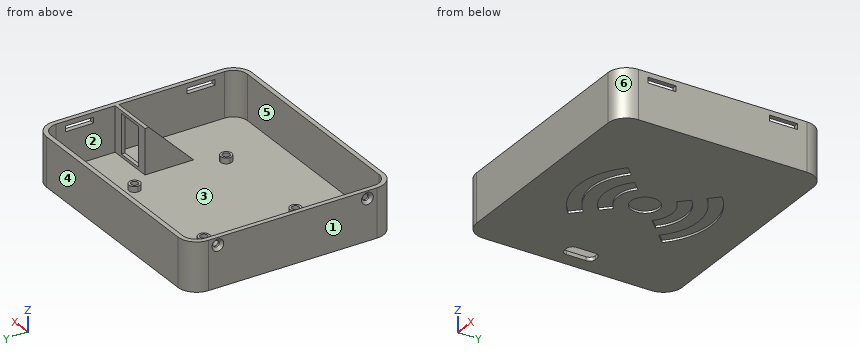
from build123d import *

# Parameters (mm, degrees)
P_IDAT_VYSUNUT_M1_DEPTH                           = 2
P_IDAT_VYSUNUT_M2_DEPTH                           = 24
SKICA6_R                                          = 3
P_IDAT_VYSUNUT_M3_DEPTH                           = 3
D_RY_PRO_KOL_K_VELIKOST_MM1_D                     = 3.8
D_RY_PRO_KOL_K_VELIKOST_MM1_DEPTH                 = 3.8
ODEBRAT_VYSUNUT_M1_DEPTH                          = 3
SKICA12_W                                         = 24
SKICA12_H                                         = 2
P_IDAT_VYSUNUT_M4_DEPTH                           = 25
P_IDAT_VYSUNUT_M5_DEPTH                           = 2
SKICA14_W                                         = 7.25
SKICA14_H                                         = 10.5
ODEBRAT_VYSUNUT_M2_DEPTH                          = 9.212713479
V_LCOV_ZAHLOUBEN_PRO_M3_ROUBY_S_PLOCH_D           = 3.4
V_LCOV_ZAHLOUBEN_PRO_M3_ROUBY_S_PLOCH_DEPTH       = 3.8
V_LCOV_ZAHLOUBEN_PRO_M3_ROUBY_S_PLOCH_CSINK_D     = 6.3
V_LCOV_ZAHLOUBEN_PRO_M3_ROUBY_S_PLOCH_CSINK_ANGLE = 90
V_LCOV_ZAHLOUBEN_PRO_M3_ROUBY_S_PLOCH_TIP         = 1.021463052
SKICA17_W                                         = 3
SKICA17_H                                         = 15
ODEBRAT_VYSUNUT_M3_DEPTH                          = 9.212713479
DUTINA1_OUTLINE_R                                 = 7.5
DUTINA1_DEPTH                                     = 1.2


# Read off the part's stored shape, not the designer's step: Dutina1
with BuildPart() as part:
    # Skica1 → Přidat vysunutím1 (new body)
    with BuildSketch(Plane.XY):
        with BuildLine():
            Line((-55, 55), (55, 55))
            ThreePointArc((55, 55), (62.071067812, 52.071067812), (65, 45))
            Line((65, 45), (65, -45))
            ThreePointArc((65, -45), (62.071067812, -52.071067812), (55, -55))
            Line((55, -55), (-55, -55))
            ThreePointArc((-55, -55), (-62.071067812, -52.071067812), (-65, -45))
            Line((-65, -45), (-65, 45))
            ThreePointArc((-65, 45), (-62.071067812, 52.071067812), (-55, 55))
        make_face()
    extrude(amount=P_IDAT_VYSUNUT_M1_DEPTH)

    # Skica2 → Přidat vysunutím2 (add)
    with BuildSketch(Plane.XY.offset(2)):
        with BuildLine():
            Line((55, 55), (-55, 55))
            ThreePointArc((-55, 55), (-62.071067812, 52.071067812), (-65, 45))
            Line((-65, 45), (-65, -45))
            ThreePointArc((-65, -45), (-62.071067812, -52.071067812), (-55, -55))
            Line((-55, -55), (55, -55))
            ThreePointArc((55, -55), (62.071067812, -52.071067812), (65, -45))
            Line((65, -45), (65, 45))
            ThreePointArc((65, 45), (62.071067812, 52.071067812), (55, 55))
        make_face()
        with BuildLine():
            Line((-55, -52.5), (55, -52.5))
            ThreePointArc((55, -52.5), (60.303300859, -50.303300859), (62.5, -45))
            Line((62.5, -45), (62.5, 45))
            ThreePointArc((62.5, 45), (60.303300859, 50.303300859), (55, 52.5))
            Line((55, 52.5), (-55, 52.5))
            ThreePointArc((-55, 52.5), (-60.303300859, 50.303300859), (-62.5, 45))
            Line((-62.5, 45), (-62.5, -45))
            ThreePointArc((-62.5, -45), (-60.303300859, -50.303300859), (-55, -52.5))
        make_face(mode=Mode.SUBTRACT)
    extrude(amount=P_IDAT_VYSUNUT_M2_DEPTH)

    # Skica6 → Přidat vysunutím3 (add)
    with BuildSketch(Plane.XY.offset(2)):
        with BuildLine():
            ThreePointArc((29, -21.5), (26.878679656, -22.378679656), (26, -24.5))
            Line((26, -24.5), (29, -24.5))
            Line((29, -24.5), (29, -21.5))
        make_face()
        with BuildLine():
            Line((29, -24.5), (26, -24.5))
            ThreePointArc((26, -24.5), (29, -27.5), (32, -24.5))
            ThreePointArc((32, -24.5), (31.121320344, -22.378679656), (29, -21.5))
            Line((29, -21.5), (29, -24.5))
        make_face()
        with BuildLine():
            ThreePointArc((26, 24.5), (26.878679656, 22.378679656), (29, 21.5))
            Line((29, 21.5), (29, 24.5))
            Line((29, 24.5), (26, 24.5))
        make_face()
        with BuildLine():
            Line((29, 24.5), (29, 21.5))
            ThreePointArc((29, 21.5), (31.121320344, 22.378679656), (32, 24.5))
            ThreePointArc((32, 24.5), (29, 27.5), (26, 24.5))
            Line((26, 24.5), (29, 24.5))
        make_face()
        with Locations((-29, 24.5)):
            Circle(SKICA6_R)
        with Locations((-29, -24.5)):
            Circle(SKICA6_R)
    extrude(amount=P_IDAT_VYSUNUT_M3_DEPTH)

    # Díry pro kolík, velikost mm1
    with Locations(Plane.XY.offset(5)):
        with Locations((29, 24.5), (29, -24.5), (-29, -24.5), (-29, 24.5)):
            Hole(D_RY_PRO_KOL_K_VELIKOST_MM1_D / 2, depth=D_RY_PRO_KOL_K_VELIKOST_MM1_DEPTH)

    # Skica11 → Odebrat vysunutím1 (cut)
    with BuildSketch(Plane.XY.offset(2)):
        with BuildLine():
            Line((-49.5, 0), (-57.5, 0))
            Line((-57.5, 0), (-57.5, -5.25))
            ThreePointArc((-57.5, -5.25), (-56.621320344, -7.371320344), (-54.5, -8.25))
            Line((-54.5, -8.25), (-52.5, -8.25))
            ThreePointArc((-52.5, -8.25), (-50.378679656, -7.371320344), (-49.5, -5.25))
            Line((-49.5, -5.25), (-49.5, 0))
        make_face()
        with BuildLine():
            Line((-57.5, 5.25), (-57.5, 0))
            Line((-57.5, 0), (-49.5, 0))
            Line((-49.5, 0), (-49.5, 5.25))
            ThreePointArc((-49.5, 5.25), (-50.378679656, 7.371320344), (-52.5, 8.25))
            Line((-52.5, 8.25), (-54.5, 8.25))
            ThreePointArc((-54.5, 8.25), (-56.621320344, 7.371320344), (-57.5, 5.25))
        make_face()
    extrude(amount=-ODEBRAT_VYSUNUT_M1_DEPTH, mode=Mode.SUBTRACT)

    # Skica12 → Přidat vysunutím4 (add)
    with BuildSketch(Plane.ZY.offset(-62.5)):
        with Locations((14, 12.5)):
            Rectangle(SKICA12_W, SKICA12_H)
    extrude(amount=P_IDAT_VYSUNUT_M4_DEPTH)

    # Skica13 → Přidat vysunutím5 (add)
    with BuildSketch(Plane.ZY.offset(-37.5)):
        Polygon((2, -12.5), (2, 11.5), (26, 11.5), align=None)
    extrude(amount=-P_IDAT_VYSUNUT_M5_DEPTH)

    # Skica14 → Odebrat vysunutím2 (cut)
    with BuildSketch(Plane(origin=(0, 13.5, 0), x_dir=(1, 0, 0), z_dir=(0, 1, 0))):
        with Locations((46.375, -8.75)):
            Rectangle(SKICA14_W, SKICA14_H)
        with Locations((53.625, -8.75)):
            Rectangle(SKICA14_W, SKICA14_H)
        with Locations((53.625, -19.25)):
            Rectangle(SKICA14_W, SKICA14_H)
        with Locations((46.375, -19.25)):
            Rectangle(SKICA14_W, SKICA14_H)
    extrude(amount=-ODEBRAT_VYSUNUT_M2_DEPTH, mode=Mode.SUBTRACT)

    # Válcové zahloubení pro M3 šrouby s plochou hlavou1
    with Locations(Plane(origin=(-65, 40, 22), x_dir=(0, 0, -1), z_dir=(-1, 0, 0))):
        with Locations((0, 0), (0, 80)):
            CounterSinkHole(V_LCOV_ZAHLOUBEN_PRO_M3_ROUBY_S_PLOCH_D / 2, V_LCOV_ZAHLOUBEN_PRO_M3_ROUBY_S_PLOCH_CSINK_D / 2, depth=V_LCOV_ZAHLOUBEN_PRO_M3_ROUBY_S_PLOCH_DEPTH, counter_sink_angle=V_LCOV_ZAHLOUBEN_PRO_M3_ROUBY_S_PLOCH_CSINK_ANGLE)
            with Locations((0, 0, -(V_LCOV_ZAHLOUBEN_PRO_M3_ROUBY_S_PLOCH_DEPTH + V_LCOV_ZAHLOUBEN_PRO_M3_ROUBY_S_PLOCH_TIP / 2))):  # 118° drill point
                Cone(0, V_LCOV_ZAHLOUBEN_PRO_M3_ROUBY_S_PLOCH_D / 2, V_LCOV_ZAHLOUBEN_PRO_M3_ROUBY_S_PLOCH_TIP, mode=Mode.SUBTRACT)

    # Skica17 → Odebrat vysunutím3 (cut)
    with BuildSketch(Plane(origin=(65, 0, 0), x_dir=(0, 0, -1), z_dir=(1, 0, 0))):
        with Locations((-22, 32.5)):
            Rectangle(SKICA17_W, SKICA17_H)
        with Locations((-22, -32.5)):
            Rectangle(SKICA17_W, SKICA17_H)
    extrude(amount=-ODEBRAT_VYSUNUT_M3_DEPTH, mode=Mode.SUBTRACT)

    # Dutina1 outline → Dutina1 (cut)
    with BuildSketch(Plane.XY):
        Circle(DUTINA1_OUTLINE_R)
        with BuildLine():
            Line((10.253048327, 10.253048327), (15.202795796, 15.202795796))
            ThreePointArc((15.202795796, 15.202795796), (0, 21.5), (-15.202795796, 15.202795796))
            Line((-15.202795796, 15.202795796), (-10.253048327, 10.253048327))
            ThreePointArc((-10.253048327, 10.253048327), (0, 14.5), (10.253048327, 10.253048327))
        make_face()
        with BuildLine():
            Line((20.152543264, 20.152543264), (25.102290732, 25.102290732))
            ThreePointArc((25.102290732, 25.102290732), (0, 35.5), (-25.102290732, 25.102290732))
            Line((-25.102290732, 25.102290732), (-20.152543264, 20.152543264))
            ThreePointArc((-20.152543264, 20.152543264), (0, 28.5), (20.152543264, 20.152543264))
        make_face()
        with BuildLine():
            ThreePointArc((-15.202795796, -15.202795796), (0, -21.5), (15.202795796, -15.202795796))
            Line((15.202795796, -15.202795796), (10.253048327, -10.253048327))
            ThreePointArc((10.253048327, -10.253048327), (0, -14.5), (-10.253048327, -10.253048327))
            Line((-10.253048327, -10.253048327), (-15.202795796, -15.202795796))
        make_face()
        with BuildLine():
            Line((-20.152543264, -20.152543264), (-25.102290732, -25.102290732))
            ThreePointArc((-25.102290732, -25.102290732), (0, -35.5), (25.102290732, -25.102290732))
            Line((25.102290732, -25.102290732), (20.152543264, -20.152543264))
            ThreePointArc((20.152543264, -20.152543264), (0, -28.5), (-20.152543264, -20.152543264))
        make_face()
    extrude(amount=DUTINA1_DEPTH, mode=Mode.SUBTRACT)


solid = part.part
Could you check a few things on this model? Use its own coordinates, in mm. Face numbers are marked on the shaded views. A direction names the side the tool comes from. Coordinates: 2 decimals unless noted, no trailing zeros. Order: outer loops, then holes, each group sorted by start corner. A loop starts at its lowest first (then second) coordinate and runs counter-clockwise, first axis right, second up.
Q1. Which directions (+Z, -Z, +X, -X, +Y, -Y) give clear straight access to the entire face, cutting with the end or side of a thin tool? Please do the marked faces 5 and 6.
Q2. Suppose I cut it at A-A on z = 9.25. Please give me the cut outline in (x, y), and give its area (3 significant figures).
Q3. Suppose I cut it at D-D on z = 22. Give the number of separate pieces and of enclosed holes in the cut face, and give its area (3 significant figures).
Q4. Will these pins go through, and if not, where does the flat tip stop? pin 1 (6 mm diameter, centred on x = 34, y = 21, fed in from +Z); pin 2 (1.1 mm diameter, centred on x = 29, y = -23.5, fed in from +Z); pin 3 (6.5 mm diameter, centred on x = -27.5, y = -25.5, fed in from +Z).
Q5. Suppose I cut it at B-B on y = 0. Please give me the cut outline in (x, z).
Q6. Thinking about a two-plate mould opening in Y: for the marked faces 1, 2, 3 and 4, which applies, released by +Y, released by -Y, zero draft, split by the parting line, or undercut?
Q7. Suppose I cut it at C-C on x = -29. Please give me the cut outline in (y, z).
Q8. Please list where these lines run through material, in increasing order: L1, parallel to X at y = 10, z = 23.75; L2, parallel to Y at x = -29, z = 2.3; L3, parallel to Y at x = 0, z = 0.45.
Answer:
1. face 5: +Z
1. face 6: +Z, -Z, +X, -Y
2. outline: (-65, -45) arc R10 ccw to (-55, -55) - (55, -55) arc R10 ccw to (65, -45) - (65, 45) arc R10 ccw to (55, 55) - (-55, 55) arc R10 ccw to (-65, 45) - close; (37.5, -5.25) - (39.5, -5.25) - (39.5, 11.5) - (42.75, 11.5) - (42.75, 13.5) - (37.5, 13.5) - close; hole (-62.5, -45) arc R7.5 ccw to (-55, -52.5) - (55, -52.5) arc R7.5 ccw to (62.5, -45) - (62.5, 11.5) - (57.25, 11.5) - (57.25, 13.5) - (62.5, 13.5) - (62.5, 45) arc R7.5 ccw to (55, 52.5) - (-55, 52.5) arc R7.5 ccw to (-62.5, 45) - close
2. area: 1,190 mm2
3. separate pieces: 5
3. enclosed holes: 0
3. area: 1,070 mm2
4. pin 1: stops at z = 2
4. pin 2: stops at z = 1.2
4. pin 3: stops at z = 5
5. outline: (-65, 0) - (-57.5, 0) - (-57.5, 2) - (-62.5, 2) - (-62.5, 26) - (-65, 26) - close; (-49.5, 0) - (-7.5, 0) - (-7.5, 1.2) - (7.5, 1.2) - (7.5, 0) - (65, 0) - (65, 26) - (62.5, 26) - (62.5, 2) - (39.5, 2) - (39.5, 14.5) - (37.5, 14.5) - (37.5, 2) - (-49.5, 2) - close
6. face 1: zero draft
6. face 2: undercut
6. face 3: undercut
6. face 4: released by +Y
7. outline: (-55, 0) - (55, 0) - (55, 26) - (52.5, 26) - (52.5, 2) - (27.5, 2) - (27.5, 5) - (26.4, 5) - (26.4, 1.2) - (22.6, 1.2) - (22.6, 5) - (21.5, 5) - (21.5, 2) - (-21.5, 2) - (-21.5, 5) - (-22.6, 5) - (-22.6, 1.2) - (-26.4, 1.2) - (-26.4, 5) - (-27.5, 5) - (-27.5, 2) - (-52.5, 2) - (-52.5, 26) - (-55, 26) - close
8. L1: x = -65 to -62.5, 37.5 to 39.5, 62.5 to 65
8. L2: y = -55 to -52.5, -27.5 to -26.4, -22.6 to -21.5, 21.5 to 22.6, 26.4 to 27.5, 52.5 to 55
8. L3: y = -55 to -35.5, -28.5 to -21.5, -14.5 to -7.5, 7.5 to 14.5, 21.5 to 28.5, 35.5 to 55
